```python
from build123d import *

# Parameters (mm, degrees)
F2_DEPTH = 11.1
F4_DEPTH = 3
F6_DEPTH = 3


# Not quite as in the source:
# - a pattern or mirror of a feature is missing from the dataset's text; its kind, count and spacing are read off the source's solid


with BuildPart() as f2:
    # F1 (on Right) → F2 (new body, symmetric)
    with BuildSketch(Plane.YZ):
        Polygon((-16, 0), (-19, 0), (-19, -29), (-10, -38), (-6, -38), (6, -38), (10.1178772148, -38), (19, -29), (19, 0), (16, 0), (16, -29), (10, -35), (0, -35), (-10, -35), (-16, -29), align=None)
    extrude(amount=F2_DEPTH, both=True)

    # F3 (on face) → F4 (join)
    with BuildSketch(Plane.YZ.offset(11.1)):
        with BuildLine():
            Line((-28, 0), (-28, -29))
            ThreePointArc((-28, -29), (-22.7279220614, -41.7279220614), (-10, -47))
            Line((-10, -47), (10, -47))
            ThreePointArc((10, -47), (22.7279220614, -41.7279220614), (28, -29))
            Line((28, -29), (28, 0))
            Line((28, 0), (19, 0))
            Line((19, 0), (19, -29))
            Line((19, -29), (10.1178772148, -38))
            Line((10.1178772148, -38), (-10, -38))
            Line((-10, -38), (-19, -29))
            Line((-19, -29), (-19, 0))
            Line((-19, 0), (-28, 0))
        make_face()
    f4 = extrude(amount=-F4_DEPTH)

    # F4_copies: F4 across plane
    add(f4.mirror(Plane(origin=(0, 0, 0), x_dir=(0, 0, -1), z_dir=(-1, 0, 0))))

    # F5 (on face) → F6 (join)
    with BuildSketch(Plane.YZ.offset(11.1)):
        Polygon((10, 0), (10, -29), (-10, -29), (-10, 0), (-16, 0), (-16, -29), (-10, -35), (0, -35), (10, -35), (16, -29), (16, 0), align=None)
    extrude(amount=-F6_DEPTH)


solid = f2.part
```
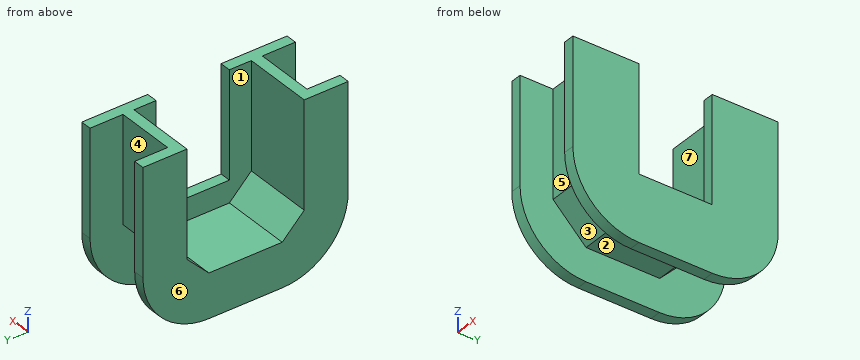
Verification items for the finished model (mm, model axes). Face numbers are marked on the shaded views. A direction names the side the tool comes from. Coordinates: 2 decimals unless noted, no trailing zeros. Loops run counter-clockwise (first coordinate to the right, second up) from the corner with the lowest first, then second, coordinate; pieces in that order, holes last. Notation, with made-up numbers: (28.5, 61.5) - (81.5, 61.5) arc R22 cw to (81.5, 99.5) - close; hole circle Ø6 at (-17, -33.75). An arc over 180 degrees is marked (long way). Return JSON: item names as keys, results as strings.
1. Tool access check on the marked faces 1, 2 and 3. Record the directions out of +Z, -Z, +X, -X, +Y, -Y that give a thin tool (end or side, any length) a straight path to the whole face; none if there is none.
Established:
{"face 1": "+Z, -X", "face 2": "-Z, +Y, -Y", "face 3": "-Z, -Y"}
2. Thickness scan on L1, parallel to X at y = -25, z = -16; L2, parallel to Y at x = 4.75, z = -17; L3, parallel to Z at x = 0.5, y = -3.5. Record the ranges inside material, lowest first.
Established:
{"L1": "x = -11.1 to -8.1, 8.1 to 11.1", "L2": "y = -19 to -16, 16 to 19", "L3": "z = -38 to -35"}
3. Section check C-C, the plane y = -23. Record the boundary of the cut face in (x, z), then the cut area to 3 significant figures.
Established:
{"outline": "(-11.1, -41.45) - (-8.1, -41.45) - (-8.1, 0) - (-11.1, 0) - close; (8.1, -41.45) - (11.1, -41.45) - (11.1, 0) - (8.1, 0) - close", "area": "249 mm2"}
4. Go/stop test with flat-tipped pins: pin 1 (5 mm diameter, centred on x = -2, y = -1.5, fed in from -Z); pin 2 (4 mm diameter, centred on x = 8.5, y = -5, fed in from +Z); pin 3 (10 mm diameter, centred on x = -0.5, z = -15.5, fed in from -Y); pin 4 (3 mm diameter, centred on x = 3.5, y = -16.5, fed in from +Z). Record where each tip stops, or that it passes through.
Established:
{"pin 1": "stops at z = -38", "pin 2": "stops at z = -29", "pin 3": "stops at y = -19", "pin 4": "stops at z = 0"}
5. Section check B-B, the plane x = -2.5. Record the boundary of the cut face in (y, z), then the cut area to 3 significant figures.
Established:
{"outline": "(-19, -29) - (-10, -38) - (10.12, -38) - (19, -29) - (19, 0) - (16, 0) - (16, -29) - (10, -35) - (-10, -35) - (-16, -29) - (-16, 0) - (-19, 0) - close", "area": "280 mm2"}
6. Section check D-D, the plane y = 3. Record the boundary of the cut face in (x, z).
Established:
{"outline": "(-11.1, -47) - (-8.1, -47) - (-8.1, -38) - (8.1, -38) - (8.1, -47) - (11.1, -47) - (11.1, -29) - (8.1, -29) - (8.1, -35) - (-11.1, -35) - close"}
7. Section check A-A, the plane z = -13. Record the boundary of the cut face in (x, y), then the cut area to 3 significant figures.
Established:
{"outline": "(-11.1, -28) - (-8.1, -28) - (-8.1, -19) - (8.1, -19) - (8.1, -28) - (11.1, -28) - (11.1, -10) - (8.1, -10) - (8.1, -16) - (-11.1, -16) - close; (-11.1, 16) - (8.1, 16) - (8.1, 10) - (11.1, 10) - (11.1, 28) - (8.1, 28) - (8.1, 19) - (-8.1, 19) - (-8.1, 28) - (-11.1, 28) - close", "area": "277 mm2"}
8. Mould release check, pull along Y, two halves, no side actions. Record for the marked faces 4, 5, 6 and 7: +Y half, -Y half, draft (parallel to the pull), parting line (faces both ways), or undercut.
Established:
{"face 4": "+Y half", "face 5": "-Y half", "face 6": "draft", "face 7": "undercut"}
